Source: three-view drawing plus pictorial views. Frame: mm from the lowest corner of the part. A direction names the side the tool comes from. Give positions to 0.01 mm unless a question says otherwise; leave off trailing zeros. Write each loop counter-clockwise with the first axis right and the second up, starting at its lowest first coordinate (ties: lowest second). Pieces come first, ordered by that corner, then holes. Notation, with made-up numbers: M 47,49.5 L 76,49.5 A14 ccw 76,67.5 Z; hole C -38,53 d9. An arc over 180 degrees is marked long. Return JSON: item names as keys, results as strings.
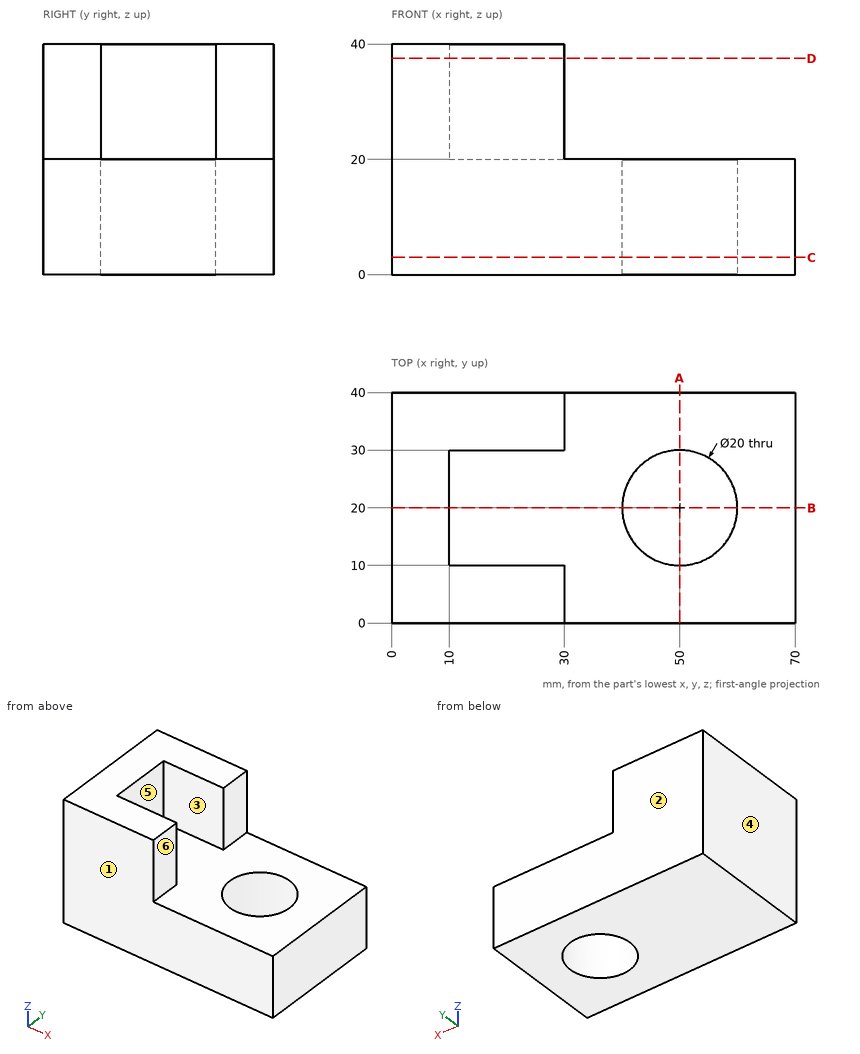
1) Cut plane D-D, the plane z = 37.5. Return the cut outline in (x, y), then the cut area to 3 significant figures.
Numbers:
{"outline": "M 0,0 L 30,0 L 30,10 L 10,10 L 10,30 L 30,30 L 30,40 L 0,40 Z", "area": "800 mm²"}
2) Draft query along Y for the marked faces 1, 2 and 3. Return one class per face: released by +Y, released by -Y, zero draft, split by the parting line, or undercut.
Numbers:
{"face 1": "released by -Y", "face 2": "released by +Y", "face 3": "undercut"}
3) Contact query for flat-ended pins moving along their axis: pin 1 Ø3 at (y, z) = (7.5, 30.5) entering from +X; pin 2 Ø6 at (x, y) = (47, 29) entering from +Z. Output: stop coordinate, or through.
Numbers:
{"pin 1": "stops at x = 30", "pin 2": "stops at z = 20"}
4) Cut plane B-B, the plane y = 20. Return the cut outline in (x, z), then the cut area to 3 significant figures.
Numbers:
{"outline": "M 0,0 L 40,0 L 40,20 L 10,20 L 10,40 L 0,40 Z; M 60,0 L 70,0 L 70,20 L 60,20 Z", "area": "1,200 mm²"}
5) Cut plane C-C, the plane z = 3. Return the cut outline in (x, y).
Numbers:
{"outline": "M 0,0 L 70,0 L 70,40 L 0,40 Z; hole C 50,20 d20"}
6) Set-up query: the marked faces 4, 5 and 6. Return all of +Z, -Z, +X, -X, +Y, -Y with unobstructed straight access to the full face (end or side cutting, diameter ignored); none if empty.
Numbers:
{"face 4": "+Z, -Z, -X, +Y, -Y", "face 5": "+Z, +X", "face 6": "+Z, +X, +Y, -Y"}
7) Cut plane A-A, the plane x = 50. Return the cut outline in (y, z), then the cut area to 3 significant figures.
Numbers:
{"outline": "M 0,0 L 10,0 L 10,20 L 0,20 Z; M 30,0 L 40,0 L 40,20 L 30,20 Z", "area": "400 mm²"}
8) Line query: line 1 (Y direction, x = 50, z = 15.25); line 2 (X direction, y = 12.5, z = 36); line 3 (Z direction, x = 56, y = 38.5). Output: solid intervals per line, ascending. Write a range as [from, to].
Numbers:
{"line 1": "y = [0, 10], [30, 40]", "line 2": "x = [0, 10]", "line 3": "z = [0, 20]"}
